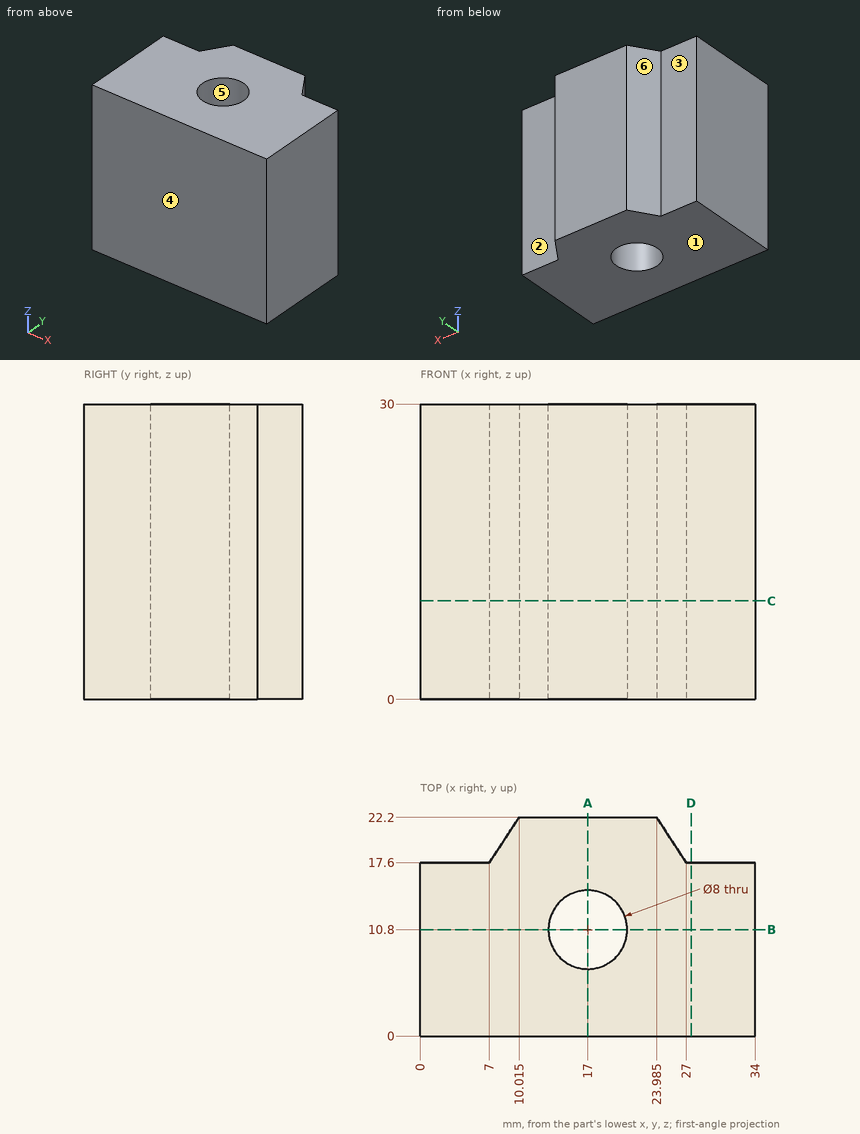
The figure shows three views and two pictorial views of one solid part (mm, origin at its lowest corner). Answer the questions. A direction names the side the tool comes from. Give positions to 0.01 mm unless a question says otherwise; leave off trailing zeros. Write each loop counter-clockwise with the first axis right and the second up, starting at its lowest first coordinate (ties: lowest second). Pieces come first, ordered by that corner, then holes. Notation, with made-up numbers: M 85,40.25 L 131,40.25 A15 cw 131,63.25 Z; hole C 85,32 d2. An arc over 180 degrees is marked long. One line per item, written item: value. Start each with the question number.
(1) Find section D-D (x = 27.5). Determine the outline of the cut face in (y, z), plus the area to 3 significant figures.
(2) Find section B-B (y = 10.8). Determine the outline of the cut face in (x, z).
(3) A flat-ended cylindrical pin translates along its axis: pin 1 Ø1.5 at (x, z) = (5, 6) entering from +Y. Find the tip coordinate at first contact, or state that the pin passes through.
(4) Find section C-C (z = 10). Determine the outline of the cut face in (x, y) (3 decimals).
(5) A tool of negligible diameter and unlimited length cuts with its end or side. For the marked faces 1, 2 and 3, from which of +Z, -Z, +X, -X, +Y, -Y can it reach the whole face along a straight path? Write none if from no direction.
(6) Find the intervals of material crossed by line 1 (Y direction, x = 17, z = 14.75); line 2 (X direction, y = 11, z = 4) (3 decimals); line 3 (Y direction, x = 16, z = 24.5), in increasing order.
(7) Determine the mould class of the marked faces 4, 5 and 6 for opening direction Y: pulls with the +Y half, pulls with the -Y half, needs draft (parallel to the pull), parting line crosses it, or undercut.
(8) Find section A-A (x = 17). Determine the outline of the cut face in (y, z).
Results below:
1. outline: M 0,0 L 17.6,0 L 17.6,30 L 0,30 Z
1. area: 528 mm^2
2. outline: M 0,0 L 13,0 L 13,30 L 0,30 Z; M 21,0 L 34,0 L 34,30 L 21,30 Z
3. pin 1: stops at y = 17.6
4. outline: M 0,0 L 34,0 L 34,17.6 L 27,17.6 L 23.985,22.2 L 10.015,22.2 L 7,17.6 L 0,17.6 Z; hole C 17,10.8 d8
5. face 1: -Z, +X, -X, +Y, -Y
5. face 2: +Z, -Z, +X, +Y
5. face 3: +Z, -Z, -X, +Y
6. line 1: y = 0 to 6.8, 14.8 to 22.2
6. line 2: x = 0 to 13.005, 20.995 to 34
6. line 3: y = 0 to 6.93, 14.67 to 22.2
7. face 4: pulls with the -Y half
7. face 5: undercut
7. face 6: pulls with the +Y half
8. outline: M 0,0 L 6.8,0 L 6.8,30 L 0,30 Z; M 14.8,0 L 22.2,0 L 22.2,30 L 14.8,30 Z
